The model under review builds one solid part; all positions refer to its coordinate system, in mm. Face numbers are marked on the shaded views. A direction names the side the tool comes from. Round coordinates to 2 decimals unless told otherwise and drop trailing zeros. Order: outer loops, then holes, each group sorted by start corner. A loop starts at its lowest first (then second) coordinate and runs counter-clockwise, first axis right, second up. Notation, with made-up numbers: (9, 25) -> (60, 25) arc R20 ccw to (60, 54) -> close; hole circle Ø11 at (80, 80). An arc over 180 degrees is marked (long way). Return JSON: item names as keys, results as strings. Group by question number.
from build123d import *

# Parameters (mm, degrees)
EXTRUDE_1_DEPTH     = 11.5
SKETCH_3_R          = 1.1
CUT_EXTRUDE_1_DEPTH = 17.6
SKETCH_6_R          = 1.1
CUT_EXTRUDE_2_DEPTH = 17.6
EXTRUDE_2_DEPTH     = 3
SKETCH_8_R          = 1.1
EXTRUDE_3_DEPTH     = 3.6
SKETCH_11_R         = 2
EXTRUDE_4_DEPTH     = 2
CHAMFER_1_SIZE      = 4
CHAMFER_1_SIZE2     = 1.865230633


with BuildPart() as part:
    # 草图1 → 凸台-拉伸1 (new body)
    with BuildSketch(Plane.XY):
        Polygon((4.65, 23), (4.65, 27.5), (3.05, 27.5), (3.05, 23), (0, 23), (0, 0), (3.05, 0), (3.05, -4.5), (4.65, -4.5), (4.65, 0), (19.65, 0), (19.65, 23), align=None)
    extrude(amount=EXTRUDE_1_DEPTH)

    # 草图3 → 切除-拉伸1 (cut, through all)
    with BuildSketch(Plane.ZY.offset(-3.05)):
        with Locations((5.75, 25.3)):
            Circle(SKETCH_3_R)
    extrude(amount=-CUT_EXTRUDE_1_DEPTH, mode=Mode.SUBTRACT)

    # 草图6 → 切除-拉伸2 (cut, through all)
    with BuildSketch(Plane.ZY.offset(-3.05)):
        with Locations((5.75, -2.3)):
            Circle(SKETCH_6_R)
    extrude(amount=-CUT_EXTRUDE_2_DEPTH, mode=Mode.SUBTRACT)

    # 草图10 → 凸台-拉伸2 (add)
    with BuildSketch(Plane.ZY):
        with BuildLine():
            Line((0.589316609, 14.714285714), (3.775477659, 8.229813665))
            ThreePointArc((3.775477659, 8.229813665), (5.75, 7), (7.724522341, 8.229813665))
            Line((7.724522341, 8.229813665), (10.910683391, 14.714285714))
            ThreePointArc((10.910683391, 14.714285714), (5.75, 23), (0.589316609, 14.714285714))
        make_face()
    extrude(amount=EXTRUDE_2_DEPTH)

    # 草图8 → 凸台-拉伸3 (add)
    with BuildSketch(Plane.ZY):
        with Locations((5.75, 9.2)):
            Circle(SKETCH_8_R)
    extrude(amount=EXTRUDE_3_DEPTH)

    # 草图11 → 凸台-拉伸4 (add)
    with BuildSketch(Plane.ZY.offset(3)):
        with Locations((5.75, 17.25)):
            Circle(SKETCH_11_R)
    extrude(amount=EXTRUDE_4_DEPTH)

    # 倒角1
    chamfer_1_edges = [part.edges().sort_by_distance(p)[0] for p in [
        (19.65, 23, 5.75),
    ]]
    chamfer_1_side = [part.faces().sort_by_distance(p)[0] for p in [
        (19.65, 11.5, 5.75),
    ]]
    chamfer(chamfer_1_edges, length=CHAMFER_1_SIZE, length2=CHAMFER_1_SIZE2, reference=chamfer_1_side[0])


solid = part.part
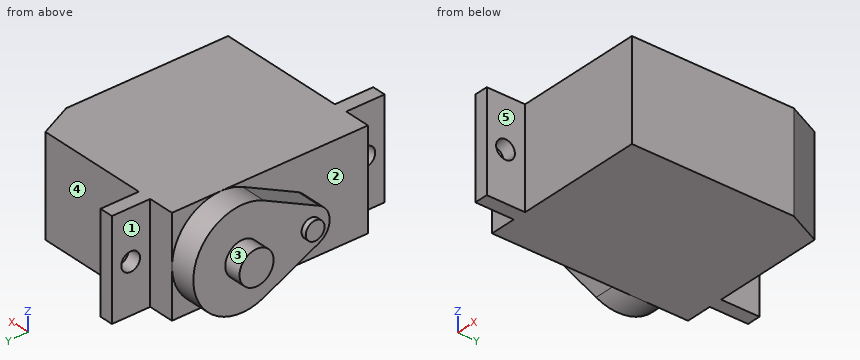
Item 1: Consider section B-B on z = 5.25. Give the number of separate pieces and of enclosed holes in the cut face, plus the area to 3 significant figures.
Item 2: Consider section D-D on y = 9.2. State the section outline as (x, z) points.
Item 3: Insertion check: pin 1 Ø3.5 at (x, z) = (1.5, 7.5) entering from +Y; pin 2 Ø1.3 at (y, z) = (-2.5, 8.5) entering from -X; pin 3 Ø1 at (y, z) = (1, 7.5) entering from -X; pin 4 Ø1.8 at (y, z) = (9.5, 6) entering from -X. Each pin has a flat end and moves straight along its axis. Give the tip position at first contact, or say it passes through.
Item 4: Consider section A-A on y = 25.3. State the section outline as (x, z) points.
Item 5: Consider section C-C on x = 7.5. State the section outline as (y, z) points, plus the area to 4 significant figures.
Item 6: For the marked faces 1, 2, 3, 4 and 5, list the 3-axis set-ups (+Z, -Z, +X, -X, +Y, -Y) from which the entire face can be reached by the end or side of a thin tool; tool diameter is ignored.
Item 7: Wall thickness on line 1 along Y through (x, z) = (3.6, 5.75); line 2 along Y through (x, z) = (2.25, 0.75); line 3 along X through (y, z) = (1.5, 6.5): over which ranges is each line inside the solid? List them lowest first.
Values:
{
 "1": {"separate pieces": "3", "enclosed holes": "0", "area": "513 mm^2"},
 "2": {"outline": "(-3.6, 4.65) -> (-3, 4.65) -> (-3, 3.3) -> (0, 3.3) -> (0, 0) -> (19.65, 0) -> (19.65, 11.5) -> (0, 11.5) -> (0, 8.2) -> (-3, 8.2) -> (-3, 6.85) -> (-3.6, 6.85) -> close"},
 "3": {"pin 1": "y = 27.5", "pin 2": "x = 3.05", "pin 3": "x = 0", "pin 4": "x = -3.6"},
 "4": {"outline": "(3.05, 0) -> (4.65, 0) -> (4.65, 4.65) -> (3.05, 4.65) -> close; (3.05, 6.85) -> (4.65, 6.85) -> (4.65, 11.5) -> (3.05, 11.5) -> close"},
 "5": {"outline": "(0, 0) -> (23, 0) -> (23, 11.5) -> (0, 11.5) -> close", "area": "264.5 mm^2"},
 "6": {"face 1": "+Z, -Z, -X, +Y", "face 2": "-X, -Y", "face 3": "-X", "face 4": "+Z, -Z, +X, +Y", "face 5": "+Z, -Z, +X, -Y"},
 "7": {"line 1": "-4.5 to -3.4, -1.2 to 24.2, 26.4 to 27.5", "line 2": "0 to 23", "line 3": "0 to 19.65"}
}
